```python
from build123d import *

# Parameters (mm, degrees)
SKETCH1_R           = 3.175
BOSS_EXTRUDE1_DEPTH = 25.4
SKETCH2_R           = 6.35
BOSS_EXTRUDE2_DEPTH = 3.175
SKETCH3_R           = 3.175
BOSS_EXTRUDE3_DEPTH = 6.35
FILLET1_R           = 1.5875
FILLET2_R           = 0.79375


with BuildPart() as part:
    # Sketch1 → Boss-Extrude1 (new body)
    with BuildSketch(Plane.XY):
        Circle(SKETCH1_R)
    extrude(amount=BOSS_EXTRUDE1_DEPTH)

    # Sketch2 → Boss-Extrude2 (add)
    with BuildSketch(Plane.XY.offset(25.4)):
        Circle(SKETCH2_R)
    extrude(amount=BOSS_EXTRUDE2_DEPTH)

    # Sketch3 → Boss-Extrude3 (add)
    with BuildSketch(Plane.XY.offset(28.575)):
        Circle(SKETCH3_R)
    extrude(amount=BOSS_EXTRUDE3_DEPTH)

    # Fillet1
    fillet1_edges = [part.edges().sort_by_distance(p)[0] for p in [
        (-3.175, 0, 34.925),
        (-3.175, 0, 0),
    ]]
    fillet(fillet1_edges, radius=FILLET1_R)

    # Fillet2
    fillet2_edges = [part.edges().sort_by_distance(p)[0] for p in [
        (-3.175, 0, 28.575),
        (-3.175, 0, 25.4),
    ]]
    fillet(fillet2_edges, radius=FILLET2_R)


solid = part.part
```
Verification items for the finished model (mm, model axes). A direction names the side the tool comes from. Give positions to 0.01 mm unless a question says otherwise; leave off trailing zeros. Order: outer loops, then holes, each group sorted by start corner. A loop starts at its lowest first (then second) coordinate and runs counter-clockwise, first axis right, second up. Notation, with made-up numbers: (2.25, 31.25) -> (55.25, 31.25) arc R23 cw to (55.25, 54.25) -> close; hole circle Ø11 at (-0.75, -27). An arc over 180 degrees is marked (long way). Use a Markdown table: item, result.
1) Tool access check on faces 1 (the cylindrical face through (-1.38, -6.2, 26.97)), 2 (the flat face through (3, 3, 25.4)), 3 (the cylindrical face through (-0.69, -3.1, 31.33)). Record the directions out of +Z, -Z, +X, -X, +Y, -Y that give a thin tool (end or side, any length) a straight path to the whole face; none if there is none.
Results:
| item | result |
|---|---|
| face 1 | +Z, -Z |
| face 2 | -Z |
| face 3 | +Z |
2) Section check A-A, the plane z = 27.5. Record the boundary of the cut face in (x, y), then the cut area to 3 significant figures.
Results:
| item | result |
|---|---|
| outline | circle Ø12.7 at (0, 0) |
| area | 127 mm² |
3) Depth check by flat-ended pin: pin 1 Ø4 at (y, z) = (0, 17.5) entering from +X (3 decimals); pin 2 Ø6 at (x, y) = (1.5, -2) entering from +Z (3 decimals); pin 3 Ø2 at (x, z) = (-3.5, 9.5) entering from +Y; pin 4 Ø3 at (x, y) = (3.5, -1) entering from +Z. Enter the tip coordinate at first touch or a pass-through.
Results:
| item | result |
|---|---|
| pin 1 | x = 3.175 |
| pin 2 | z = 34.925 |
| pin 3 | y = 1.96 |
| pin 4 | z = 34.83 |
4) Section check B-B, the plane z = 20. Record the boundary of the cut face in (x, y) (3 decimals), then the cut area to 3 significant figures.
Results:
| item | result |
|---|---|
| outline | circle Ø6.35 at (0, 0) |
| area | 31.7 mm² |
5) Section check C-C, the plane y = -4.5. Record the boundary of the cut face in (x, z) (3 decimals), then the cut area to 3 significant figures.
Results:
| item | result |
|---|---|
| outline | (-4.48, 25.4) -> (4.48, 25.4) -> (4.48, 28.575) -> (-4.48, 28.575) -> close |
| area | 28.4 mm² |
6) Material ranges on probe 1 along Z at (x, y) = (0.5, 4.75) (3 decimals); probe 2 along X at (y, z) = (-0.75, 29); probe 3 along X at (y, z) = (-2.75, 3), recorded low to high.
Results:
| item | result |
|---|---|
| probe 1 | 25.4 to 28.575 |
| probe 2 | -3.18 to 3.18 |
| probe 3 | -1.59 to 1.59 |
